Solid Edge part; units mm, degrees
sketch "Sketch1" plane through (0, 0, 0) normal (0, 0, 1) x (1, 0, 0)
  line L0 (-2.5, 0) -> (-2.5, 3)
  line L1 (-2.5, 3) -> (2.5, 3)
  line L2 (2.5, 3) -> (2.5, 4)
  line L3 (2.5, 4) -> (3.5, 4)
  line L4 (3.5, 4) -> (3.5, 3)
  line L5 (3.5, 3) -> (10.8865, 3)
  line L6 (10.8865, 3) -> (11.5, 2.3865)
  line L7 (11.5, 2.3865) -> (11.5, 0)
  line L8 (11.5, 0) -> (-2.5, 0)
revolve "RevolvedProtrusion1" add sketch "Sketch1" angle 360 about axis through (11.5, 0, 0) along (-1, 0, 0)
cosmetic_thread "Thread1"
sketch "Sketch2" plane through (0, 0, 0) normal (0, 0, 1) x (1, 0, 0)
  line L0 (-2.5, 0) -> (-2.5, 1.7321)
  line L1 (-2.5, 1.7321) -> (-1.5, 0)
  line L2 (-1.5, 0) -> (-2.5, 0)
revolve "RevolvedCutout1" cut sketch "Sketch2" angle 360 about axis through (-1.5, 0, 0) along (-1, 0, 0)
sketch "Sketch3" plane through (-2.5, 0, 0) normal (1, 0, 0) x (0, 1, 0)
  line L0 (0.866, 1.5) -> (-0.866, 1.5)
  line L1 (-0.866, 1.5) -> (-1.7321, 0)
  line L2 (-1.7321, 0) -> (-0.866, -1.5)
  line L3 (-0.866, -1.5) -> (0.866, -1.5)
  line L4 (0.866, -1.5) -> (1.7321, 0)
  line L5 (1.7321, 0) -> (0.866, 1.5)
extrude "ExtrudedCutout_1" cut sketch "Sketch3" along normal blind 1.7857
sketch "Sketch4" plane through (0, 0, 0) normal (0, 0, 1) x (1, 0, 0)
  line L0 (-0.7143, 0) -> (-0.7143, 1.7321)
  line L1 (-0.7143, 1.7321) -> (0.2857, 0)
  line L2 (0.2857, 0) -> (-0.7143, 0)
revolve "RevolvedCutout2" cut sketch "Sketch4" angle 360 about axis through (0.2857, 0, 0) along (-1, 0, 0)
properties material "Steel"
Build history of the part. All positions in model axes, mm. A direction names the side the tool comes from. Coordinates: 2 decimals unless noted, no trailing zeros.
(1) Mould opens along Y. For faces 1 (the flat face through (-1.62, 1.305, 0.74)), 2 (the cylindrical face through (7, -3, 0)), 3 (the flat face through (2.5, 1, -3)) say: pulls with the +Y half, pulls with the -Y half, needs draft (parallel to the pull), parting line crosses it, or undercut.
(2) 3-axis set-ups, long thin cutter, end or side, ignore diameter. For faces 4 (the cylindrical face through (0, -3, 0)), 5 (the cylindrical face through (3.007, -0.867, -3.905)), 6 (the flat face through (3.5, 1, -3)): which of +Z, -Z, +X, -X, +Y, -Y reach the whole face in a straight line?
(3) Drill centre lines: line 1 (X direction, y = 2.75, z = -2); line 2 (Z direction, x = -2, y = -0.75); line 3 (X direction, y = -0.5, z = 0). Where is each one in solid material? Low to high.
(4) Pin check, flat tips, straight feed: pin 1 Ø1 at (y, z) = (-3, -3) entering from -X; pin 2 Ø1 at (x, y) = (3, -1) entering from +Z; pin 3 Ø1.9 at (x, y) = (-2, 0) entering from -Z. Stop position of each tip, or through.
Working result:
1. face 1: undercut
1. face 2: parting line crosses it
1. face 3: needs draft
2. face 4: -X
2. face 5: +X, -X
2. face 6: +X
3. line 1: x = 2.5 to 3.5
3. line 2: z = -2.9 to -1.5, 1.5 to 2.9
3. line 3: x = 0 to 11.5
4. pin 1: stops at x = 2.5
4. pin 2: stops at z = 3.97
4. pin 3: stops at z = -3
